from build123d import *

# Parameters (mm, degrees)
F0_W     = 64.246036
F0_H     = 62.718913
F2_DEPTH = 25.4
F3_R     = 5.08
F4_SIZE  = 5.08
F5_D     = 5


with BuildPart() as f2:
    # F0 (on Top) → F2 (new body)
    with BuildSketch(Plane.XY):
        with Locations((-32.123018, 31.359457)):
            Rectangle(F0_W, F0_H)
    extrude(amount=F2_DEPTH)

    # F3
    f3_edges = [f2.edges().sort_by_distance(p)[0] for p in [
        (0, 0, 12.7),
    ]]
    fillet(f3_edges, radius=F3_R)

    # F4
    f4_edges = [f2.edges().sort_by_distance(p)[0] for p in [
        (0, 33.899456, 25.4),
    ]]
    chamfer(f4_edges, length=F4_SIZE)

    # F5 (through all)
    with Locations(Plane(origin=(0, 0, 0), x_dir=(1, 0, 0), z_dir=(0, 0, -1))):
        with Locations((-6.916952, 0)):
            Hole(F5_D / 2)


solid = f2.part
Verification items for the finished model (mm, model axes). Round coordinates to 2 decimals unless told otherwise and drop trailing zeros. Loops run counter-clockwise (first coordinate to the right, second up) from the corner with the lowest first, then second, coordinate; pieces in that order, holes last. Notation, with made-up numbers: (-33.75, 7.25) - (-5.75, 7.25) arc R9 ccw to (-5.75, 15.25) - close; hole circle Ø3 at (17.25, 82). An arc over 180 degrees is marked (long way). Answer in a Markdown table with one row per item. Add a question column.
Q1. Material ranges on line 1 (Y direction, x = -5, z = 11.25); line 2 (Z direction, x = -5, y = 39); line 3 (Y direction, x = -58, z = 21.75), recorded low to high.
Q2. Section check A-A on x = -8. Enter the section's corners in (y, z).
Q3. Release check for a two-part mould opening along X. For faces 1 (the face through (0, 33, 10)), 2 (the face through (-6.9, 2.5, 11.6)), 3 (the face through (-33, 32, 0)) record: pulls with the +X half, pulls with the -X half, needs draft (parallel to the pull), parting line crosses it, or undercut.
Found:
| question | item | result |
|---|---|---|
| 1 | line 1 | y = 1.6 to 62.72 |
| 1 | line 2 | z = 0 to 25.32 |
| 1 | line 3 | y = 1.43 to 62.72 |
| 2 | outline | (2.25, 0) - (62.72, 0) - (62.72, 25.4) - (5.08, 25.4) - (2.25, 22.57) - close |
| 3 | face 1 | pulls with the +X half |
| 3 | face 2 | undercut |
| 3 | face 3 | needs draft |
